Geometry check sheet. Reference: the model listing, model coordinates, mm. Round coordinates to 2 decimals unless told otherwise and drop trailing zeros. Write each loop counter-clockwise with the first axis right and the second up, starting at its lowest first coordinate (ties: lowest second). Pieces come first, ordered by that corner, then holes.
Item 1: Cross-section at A-A (x = -37). Enter the section's corners in (y, z), then the cut area to 3 significant figures.
Item 2: Cross-section at C-C (z = 1.5). Enter the section's corners in (x, y).
Item 3: Cross-section at B-B (y = 3.75). Enter the section's corners in (x, z).
Item 4: Scan lines: probe 1 along Y at (x, z) = (-7, 1.6); probe 2 along Y at (x, z) = (-69.5, 2.7); probe 3 along X at (y, z) = (-5.5, 1.7). Record each from-to range of solid material in increasing order.
Item 5: Depth check by flat-ended pin: P1, Ø1.8, axis at x = 37, y = 0, coming from the -Z side; P2, Ø1, axis at y = 6, z = 2.5, coming from the +X side. Enter the tip coordinate at first touch or a pass-through.
Item 6: Cross-section at D-D (y = 9.75). Enter the section's corners in (x, z), then the cut area to 3 significant figures.
from build123d import *

# Parameters (mm, degrees)
ESQUISSE1_R        = 1.5
ESQUISSE1_R_2      = 6.5
BOSS_EXTRU_1_DEPTH = 3


with BuildPart() as part:
    # Esquisse1 → Boss.-Extru.1 (new body)
    with BuildSketch(Plane.XY):
        with BuildLine():
            Line((-70, 12), (70, 12))
            ThreePointArc((70, 12), (82, 0), (70, -12))
            Line((70, -12), (-70, -12))
            ThreePointArc((-70, -12), (-82, 0), (-70, 12))
        make_face()
        with Locations((-7, 0)):
            Circle(ESQUISSE1_R, mode=Mode.SUBTRACT)
        with Locations((-70, 0)):
            Circle(ESQUISSE1_R, mode=Mode.SUBTRACT)
        with Locations(Location((70, 0, 0), (0, 0, 180))):
            Circle(ESQUISSE1_R_2, mode=Mode.SUBTRACT)
        with Locations((-37, 0)):
            Circle(ESQUISSE1_R, mode=Mode.SUBTRACT)
        with Locations((37, 0)):
            Circle(ESQUISSE1_R, mode=Mode.SUBTRACT)
    extrude(amount=BOSS_EXTRU_1_DEPTH)


solid = part.part
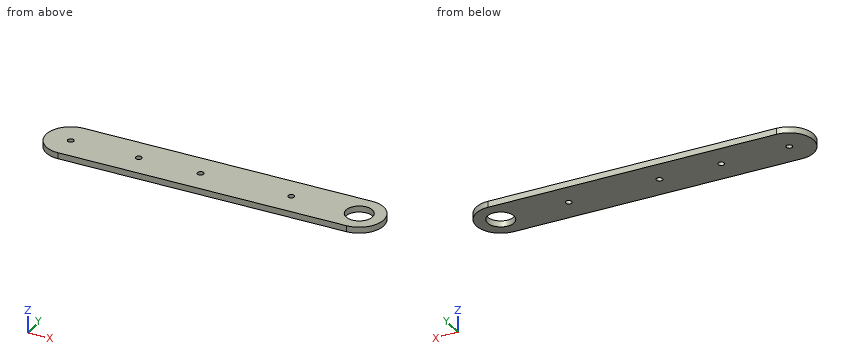
Resolved:
1. outline: (-12, 0) - (-1.5, 0) - (-1.5, 3) - (-12, 3) - close; (1.5, 0) - (12, 0) - (12, 3) - (1.5, 3) - close
1. area: 63.0 mm2
2. outline: (-70, -12) - (70, -12) arc R12 ccw to (70, 12) - (-70, 12) arc R12 ccw to start; hole circle Ø3 at (-70, 0); hole circle Ø3 at (-37, 0); hole circle Ø3 at (-7, 0); hole circle Ø3 at (37, 0); hole circle Ø13 at (70, 0)
3. outline: (-81.4, 0) - (64.69, 0) - (64.69, 3) - (-81.4, 3) - close; (75.31, 0) - (81.4, 0) - (81.4, 3) - (75.31, 3) - close
4. probe 1: y = -12 to -1.5, 1.5 to 12
4. probe 2: y = -12 to -1.41, 1.41 to 12
4. probe 3: x = -80.67 to 66.54, 73.46 to 80.67
5. P1: passes through
5. P2: stops at x = 80.67
6. outline: (-77, 0) - (77, 0) - (77, 3) - (-77, 3) - close
6. area: 462 mm2
